```python
from build123d import *

# Parameters (mm, degrees)
SKETCH1_R           = 38
BOSS_EXTRUDE1_DEPTH = 24
FILLET1_R           = 8.89
SKETCH4_R           = 10.922
BOSS_EXTRUDE2_DEPTH = 3.302
CUT_EXTRUDE3_DEPTH  = 17.526


with BuildPart() as part:
    # Sketch1 → Boss-Extrude1 (new body)
    with BuildSketch(Plane(origin=(0, 0, 0), x_dir=(0, 0, -1), z_dir=(1, 0, 0))):
        Circle(SKETCH1_R)
    extrude(amount=BOSS_EXTRUDE1_DEPTH)

    # Fillet1
    fillet1_edges = [part.edges().sort_by_distance(p)[0] for p in [
        (0, 0, 38),
        (24, 0, 38),
    ]]
    fillet(fillet1_edges, radius=FILLET1_R)

    # Sketch4 → Boss-Extrude2 (add)
    with BuildSketch(Plane.ZY):
        with Locations(Location((0, 0, 0), (0, 0, 180))):
            Circle(SKETCH4_R)
    extrude(amount=BOSS_EXTRUDE2_DEPTH)

    # Sketch5 → Cut-Extrude3 (cut)
    with BuildSketch(Plane.ZY.offset(3.302)):
        with BuildLine():
            Line((-1.658312395, 2.5), (1.658312395, 2.5))
            ThreePointArc((1.658312395, 2.5), (0, -3), (-1.658312395, 2.5))
        make_face()
    extrude(amount=-CUT_EXTRUDE3_DEPTH, mode=Mode.SUBTRACT)


solid = part.part
```
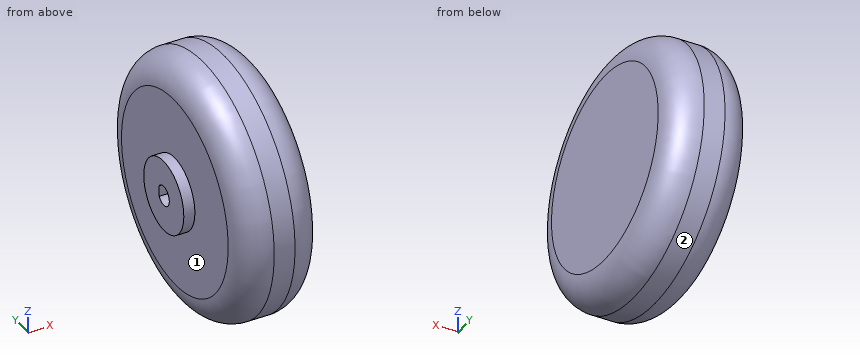
The model under review builds one solid part; all positions refer to its coordinate system, in mm. Face numbers are marked on the shaded views. A direction names the side the tool comes from. Round coordinates to 2 decimals unless told otherwise and drop trailing zeros. Loops run counter-clockwise (first coordinate to the right, second up) from the corner with the lowest first, then second, coordinate; pieces in that order, holes last. Notation, with made-up numbers: (-18.5, -7) -> (-5.5, -7) arc R26 cw to (-5.5, 16) -> close; hole circle Ø2 at (-6.5, 66.25). An arc over 180 degrees is marked (long way). Answer as a JSON object with one key per item and string values. Group by question number.
1) We need section B-B on z = 0. Write out the cut boundary in (x, y), then the cut area to 3 significant figures.
2) We need section C-C on x = 17.75. Write out the cut boundary in (y, z).
3) We need section A-A on y = 0. Write out the cut boundary in (x, z).
4) For pin 1 Ø6 at (y, z) = (-12, 29.5) entering from -X; pin 2 Ø12 at (x, z) = (0.5, 11) entering from -Y; pin 3 Ø1.7 at (x, z) = (2.5, 0) entering from -Y, all flat-tipped, find the tip position at first contact; note any pin that passes through.
5) For the marked faces 1 and 2, list the 3-axis set-ups (+Z, -Z, +X, -X, +Y, -Y) from which the entire face can be reached by the end or side of a thin tool; tool diameter is ignored.
6) For line 1 (Y direction, x = 6.5, z = 0); line 2 (X direction, y = -10, z = 17); line 3 (X direction, y = 1, z = 1), list the stretches that pass through material, from the lowest coordinate up. Write a range as [from, to].
Result set:
{
 "1": {"outline": "(-3.3, -10.92) -> (0, -10.92) -> (0, -29.11) arc R8.89 ccw to (8.89, -38) -> (15.11, -38) arc R8.89 ccw to (24, -29.11) -> (24, 29.11) arc R8.89 ccw to (15.11, 38) -> (8.89, 38) arc R8.89 ccw to (0, 29.11) -> (0, 10.92) -> (-3.3, 10.92) -> (-3.3, 2.5) -> (14.22, 2.5) -> (14.22, -3) -> (-3.3, -3) -> close", "area": "1,730 mm²"},
 "2": {"outline": "circle Ø75.2 at (0, 0)"},
 "3": {"outline": "(-3.3, -10.92) -> (0, -10.92) -> (0, -29.11) arc R8.89 ccw to (8.89, -38) -> (15.11, -38) arc R8.89 ccw to (24, -29.11) -> (24, 29.11) arc R8.89 ccw to (15.11, 38) -> (8.89, 38) arc R8.89 ccw to (0, 29.11) -> (0, 10.92) -> (-3.3, 10.92) -> (-3.3, 3) -> (14.22, 3) -> (14.22, -3) -> (-3.3, -3) -> close"},
 "4": {"pin 1": "x = 0", "pin 2": "y = -36.54", "pin 3": "y = -36.06"},
 "5": {"face 1": "-X", "face 2": "+X, -X"},
 "6": {"line 1": "[-37.67, -3], [2.5, 37.67]", "line 2": "[0, 24]", "line 3": "[14.22, 24]"}
}
